Read the model definition and answer for the solid it produces. Units are mm, in the model's axes. A direction names the side the tool comes from. Give positions to 0.01 mm unless a question says otherwise; leave off trailing zeros. Write each loop counter-clockwise with the first axis right and the second up, starting at its lowest first coordinate (ties: lowest second). Pieces come first, ordered by that corner, then holes.
```python
from build123d import *

# Parameters (mm, degrees)
SKETCH_1_W          = 74
SKETCH_1_H          = 43
EXTRUDE_1_DEPTH     = 30
EXTRUDE_4_DEPTH     = 74
CUT_EXTRUDE_2_REACH = 115.492
SKETCH_8_W          = 67
SKETCH_8_H          = 67
SKETCH_10_W         = 70.8
SKETCH_10_H         = 32.499098008
CUT_EXTRUDE_3_DEPTH = 18
CUT_EXTRUDE_5_REACH = 114.206
SKETCH_11_W         = 67
SKETCH_11_H         = 1.389705156
SKETCH_12_W         = 5
SKETCH_12_H         = 5
SKETCH_12_R         = 1.5
EXTRUDE_6_DEPTH     = 18
CHAMFER_1_SIZE      = 1


with BuildPart() as part:
    # 草图1 → 凸台-拉伸1 (new body)
    with BuildSketch(Plane(origin=(0, 0, 0), x_dir=(1, 0, 0), z_dir=(0, 1, 0))):
        Rectangle(SKETCH_1_W, SKETCH_1_H)
    extrude(amount=EXTRUDE_1_DEPTH)

    # 草图7 → 凸台-拉伸4 (add, through all)
    with BuildSketch(Plane.ZY.offset(37)):
        Polygon((21.5, 30), (15.399098008, 99.733628866), (14.199098008, 99.733628866), (14.199098008, 30), align=None)
    extrude(amount=-EXTRUDE_4_DEPTH)

    # 切除-拉伸2: up to this plane
    cut_extrude_2_end = Plane(origin=(37, 99.733628866, 14.199098008), z_dir=(0, 0, -1))
    # 草图8 → 切除-拉伸2 (cut, up to the surface)
    with BuildSketch(Plane(origin=(0, 1.990014723, 22.745972372), x_dir=(1, 0, 0), z_dir=(0, 0.08715574274766194, 0.9961946980917453)), mode=Mode.PRIVATE) as cut_extrude_2_sk1:
        with Locations((0, 63.011992474)):
            Rectangle(SKETCH_8_W, SKETCH_8_H)
    cut_extrude_2_tool1 = split(extrude(cut_extrude_2_sk1.sketch, amount=-CUT_EXTRUDE_2_REACH, mode=Mode.PRIVATE), bisect_by=cut_extrude_2_end, keep=Keep.BOTH, mode=Mode.PRIVATE)
    add(cut_extrude_2_tool1.solids().sort_by_distance((0, 64.762228, 17.254115))[0], mode=Mode.SUBTRACT)

    # 草图10 → 切除-拉伸3 (cut)
    with BuildSketch(Plane(origin=(0, 30, 0), x_dir=(1, 0, 0), z_dir=(0, 1, 0))):
        with Locations((0, 3.650450996)):
            Rectangle(SKETCH_10_W, SKETCH_10_H)
    extrude(amount=-CUT_EXTRUDE_3_DEPTH, mode=Mode.SUBTRACT)

    # 切除-拉伸5: up to this face of the body (flat: up to its plane)
    cut_extrude_5_end = Plane(part.part.faces().sort_by_distance((0, 64.762227542, 17.254115366))[0])
    # 草图11 → 切除-拉伸5 (cut, up to the picked face)
    with BuildSketch(Plane(origin=(0, 0, 14.199098008), x_dir=(-1, 0, 0), z_dir=(0, 0, -1)), mode=Mode.PRIVATE) as cut_extrude_5_sk1:
        with Locations((0, 30.694852578)):
            Rectangle(SKETCH_11_W, SKETCH_11_H)
    cut_extrude_5_tool1 = split(extrude(cut_extrude_5_sk1.sketch, amount=-CUT_EXTRUDE_5_REACH, mode=Mode.PRIVATE), bisect_by=cut_extrude_5_end, keep=Keep.BOTH, mode=Mode.PRIVATE)
    add(cut_extrude_5_tool1.solids().sort_by(Axis((0, 30.694853, 14.199098), (0, 0, 1)))[0], mode=Mode.SUBTRACT)

    # 草图12 → 凸台-拉伸6 (add)
    # profile 1 of 4: a face of its own
    with BuildSketch(Plane(origin=(0, 12, 0), x_dir=(1, 0, 0), z_dir=(0, 1, 0))):
        with Locations((-32.9, 17.4)):
            Rectangle(SKETCH_12_W, SKETCH_12_H)
        with Locations(Location((-32.904560765, 17.513886845, 0), (0, 0, 90))):
            Circle(SKETCH_12_R, mode=Mode.SUBTRACT)
    # profile 2 of 4: a face of its own
    with BuildSketch(Plane(origin=(0, 12, 0), x_dir=(1, 0, 0), z_dir=(0, 1, 0))):
        with Locations((32.9, 17.4)):
            Rectangle(SKETCH_12_W, SKETCH_12_H)
        with Locations(Location((32.9, 17.4, 0), (0, 0, 90))):
            Circle(SKETCH_12_R, mode=Mode.SUBTRACT)
    # profile 3 of 4: a face of its own
    with BuildSketch(Plane(origin=(0, 12, 0), x_dir=(1, 0, 0), z_dir=(0, 1, 0))):
        with Locations((-32.9, -10.099098008)):
            Rectangle(SKETCH_12_W, SKETCH_12_H)
        with Locations(Location((-32.9, -10.099098008, 0), (0, 0, 90))):
            Circle(SKETCH_12_R, mode=Mode.SUBTRACT)
    # profile 4 of 4: a face of its own
    with BuildSketch(Plane(origin=(0, 12, 0), x_dir=(1, 0, 0), z_dir=(0, 1, 0))):
        with Locations((32.9, -10.099098008)):
            Rectangle(SKETCH_12_W, SKETCH_12_H)
        with Locations(Location((32.9, -10.099098008, 0), (0, 0, 90))):
            Circle(SKETCH_12_R, mode=Mode.SUBTRACT)
    extrude(amount=EXTRUDE_6_DEPTH)

    # 倒角1
    # the kernel refuses this chamfer: 1 mm, written as the material it takes off along each edge
    with BuildSketch(Plane(origin=(37, -2.571682988, 21.5), x_dir=(0, 0, -1), z_dir=(0, 1, 0))) as chamfer_1_piece_1:
        Polygon((CHAMFER_1_SIZE, 0), (0, CHAMFER_1_SIZE), (0, 0), align=None)
    extrude(amount=45.430097928, mode=Mode.SUBTRACT)
    with BuildSketch(Plane(origin=(-37, -2.571682988, 21.5), x_dir=(0, 0, -1), z_dir=(0, 1, 0))) as chamfer_1_piece_2:
        Polygon((CHAMFER_1_SIZE, 0), (0, -CHAMFER_1_SIZE), (0, 0), align=None)
    extrude(amount=45.430097928, mode=Mode.SUBTRACT)
    with BuildSketch(Plane(origin=(-37, -2.571682988, -21.5), x_dir=(1, 0, 0), z_dir=(0, 1, 0))) as chamfer_1_piece_3:
        Polygon((CHAMFER_1_SIZE, 0), (0, -CHAMFER_1_SIZE), (0, 0), align=None)
    extrude(amount=35.143365976, mode=Mode.SUBTRACT)
    with BuildSketch(Plane(origin=(37, -2.571682988, -21.5), x_dir=(-1, 0, 0), z_dir=(0, 1, 0))) as chamfer_1_piece_4:
        Polygon((CHAMFER_1_SIZE, 0), (0, CHAMFER_1_SIZE), (0, 0), align=None)
    extrude(amount=35.143365976, mode=Mode.SUBTRACT)


solid = part.part
```
Item 1: Find the intervals of material crossed by line 1 along Z through (x, y) = (-32.9, 25.75); line 2 along X through (y, z) = (16.75, -17.4); line 3 along Z through (x, y) = (32.9, 25.75), in increasing order.
Result set:
line 1: z = -21.5 to -19.01, -16.01 to -14.9, 7.6 to 8.6, 11.6 to 21.5
line 2: x = -37 to -34.4, -31.41 to -30.4, 30.4 to 31.4, 34.4 to 37
line 3: z = -21.5 to -18.9, -15.9 to -14.9, 7.6 to 8.6, 11.6 to 21.5
Item 2: Section D-D (z = -17.4) is taken. Write down the section's boundary in (x, y).
Result set:
outline: (-37, 0) - (37, 0) - (37, 30) - (34.4, 30) - (34.4, 12) - (31.4, 12) - (31.4, 30) - (30.4, 30) - (30.4, 12) - (-30.4, 12) - (-30.4, 30) - (-31.41, 30) - (-31.41, 12) - (-34.4, 12) - (-34.4, 30) - (-37, 30) - close
Item 3: Section B-B (x = -11) is taken. Write down the section's boundary in (y, z), and give its area (3 significant figures).
Result set:
outline: (0, -21.5) - (30, -21.5) - (30, -19.9) - (12, -19.9) - (12, 12.6) - (30, 12.6) - (30, 20.3) - (98.13, 14.33) - (98.12, 14.2) - (99.73, 14.2) - (99.73, 15.4) - (30, 21.5) - (0, 21.5) - close
area: 789 mm2
Item 4: Which of the six approach directions +Z, -Z, +X, -X, +Y, -Y give full straight-line access (tool end or side, diameter ignored) to faces 5 (the flat face through (37, 17, 0)), 6 (the flat face through (3, 30, 13)), 7 (the flat face through (0, 21, -19.9))?
Result set:
face 5: +Z, -Z, +X, +Y, -Y
face 6: -Z
face 7: +Y
Item 5: Section A-A (z = -5.5) is taken. Write down the section's boundary in (x, y), and give its area (3 significant figures).
Result set:
outline: (-37, 0) - (37, 0) - (37, 30) - (35.4, 30) - (35.4, 12) - (-35.4, 12) - (-35.4, 30) - (-37, 30) - close
area: 946 mm2
Item 6: Section C-C (y = 76) is taken. Write down the section's boundary in (x, z), and give its area (3 significant figures).
Result set:
outline: (-37, 14.2) - (-33.5, 14.2) - (-33.5, 16.27) - (33.5, 16.27) - (33.5, 14.2) - (37, 14.2) - (37, 17.48) - (-37, 17.48) - close
area: 104 mm2
Item 7: Determine the mould class of faces 1 (the flat face through (-0.469, 63.59, 17.357)), 2 (the flat face through (-33, 21, 7.599)), 3 (the flat face through (33, 12, -17)), 4 (the flat face through (-1, 0, 0)) for opening direction Z: pulls with the +Z half, pulls with the -Z half, needs draft (parallel to the pull), parting line crosses it, or undercut.
Result set:
face 1: pulls with the -Z half
face 2: undercut
face 3: undercut
face 4: needs draft
Item 8: Each of these flat-tipped pins is pushed along its axis until it touches: pin 1 Ø3 at (x, y) = (10, 36) entering from +Z; pin 2 Ø12.5 at (x, z) = (3, 7) entering from +Y; pin 3 Ø3 at (x, y) = (-4.5, 66) entering from +Z. Where does it stop, or does it pass through?
Result set:
pin 1: stops at z = 21.11
pin 2: stops at y = 30
pin 3: stops at z = 18.48
